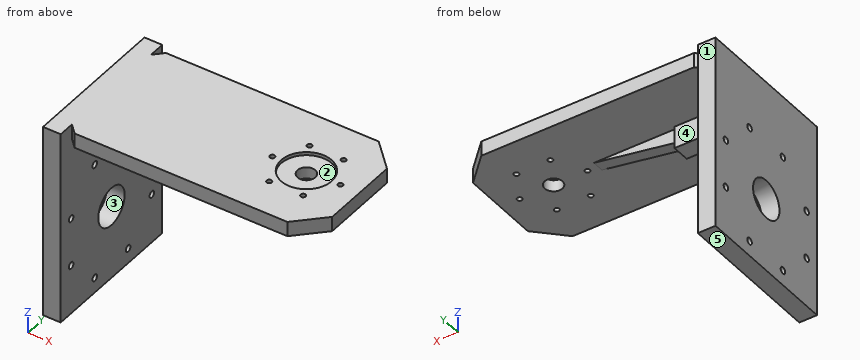
from build123d import *

# Parameters (mm, degrees)
SK_TOP_PLATE_R         = 1.7
SK_TOP_PLATE_R_2       = 6
TOP_PLATE_DEPTH        = 10
SK_YAW_PILOT_RECESS_R  = 17.15
YAW_PILOT_RECESS_DEPTH = 2.2
SK_BACK_PLATE_W        = 132
SK_BACK_PLATE_H        = 100
SK_BACK_PLATE_R        = 2.25
SK_BACK_PLATE_R_2      = 13
BACK_PLATE_DEPTH       = 12
RIB_DEPTH              = 8
SK_KEEL_W              = 58
SK_KEEL_H              = 15
KEEL_DEPTH             = 12


with BuildPart() as part:
    # SK_Top_Plate → Top_Plate (new body)
    with BuildSketch(Plane.XY.offset(72)):
        Polygon((-126, -45), (18, -45), (36, -27), (36, 27), (18, 45), (-126, 45), (-144, 27), (-144, -27), align=None)
        with Locations((23, 0)):
            Circle(SK_TOP_PLATE_R, mode=Mode.SUBTRACT)
        with Locations((11.5, 19.918584287)):
            Circle(SK_TOP_PLATE_R, mode=Mode.SUBTRACT)
        with Locations((-11.5, 19.918584287)):
            Circle(SK_TOP_PLATE_R, mode=Mode.SUBTRACT)
        with Locations((-23, 0)):
            Circle(SK_TOP_PLATE_R, mode=Mode.SUBTRACT)
        with Locations((-11.5, -19.918584287)):
            Circle(SK_TOP_PLATE_R, mode=Mode.SUBTRACT)
        with Locations((11.5, -19.918584287)):
            Circle(SK_TOP_PLATE_R, mode=Mode.SUBTRACT)
        Circle(SK_TOP_PLATE_R_2, mode=Mode.SUBTRACT)
    extrude(amount=TOP_PLATE_DEPTH)

    # SK_Yaw_Pilot_Recess → Yaw_Pilot_Recess (cut)
    with BuildSketch(Plane.XY.offset(82)):
        Circle(SK_YAW_PILOT_RECESS_R)
    extrude(amount=-YAW_PILOT_RECESS_DEPTH, mode=Mode.SUBTRACT)

    # SK_Back_Plate → Back_Plate (add)
    with BuildSketch(Plane(origin=(-144, 0, 0), x_dir=(0, 0, -1), z_dir=(1, 0, 0))):
        with Locations((-16, 0)):
            Rectangle(SK_BACK_PLATE_W, SK_BACK_PLATE_H)
        with Locations((39.726819898, 16.455387592)):
            Circle(SK_BACK_PLATE_R, mode=Mode.SUBTRACT)
        with Locations((16.455387592, 39.726819898)):
            Circle(SK_BACK_PLATE_R, mode=Mode.SUBTRACT)
        with Locations((-16.455387592, 39.726819898)):
            Circle(SK_BACK_PLATE_R, mode=Mode.SUBTRACT)
        with Locations((-39.726819898, 16.455387592)):
            Circle(SK_BACK_PLATE_R, mode=Mode.SUBTRACT)
        with Locations((-39.726819898, -16.455387592)):
            Circle(SK_BACK_PLATE_R, mode=Mode.SUBTRACT)
        with Locations((-16.455387592, -39.726819898)):
            Circle(SK_BACK_PLATE_R, mode=Mode.SUBTRACT)
        with Locations((16.455387592, -39.726819898)):
            Circle(SK_BACK_PLATE_R, mode=Mode.SUBTRACT)
        with Locations((39.726819898, -16.455387592)):
            Circle(SK_BACK_PLATE_R, mode=Mode.SUBTRACT)
        Circle(SK_BACK_PLATE_R_2, mode=Mode.SUBTRACT)
    extrude(amount=BACK_PLATE_DEPTH)

    # SK_Rib → Rib (add)
    with BuildSketch(Plane(origin=(0, -4, 0), x_dir=(1, 0, 0), z_dir=(0, 1, 0))):
        Polygon((-144, -52), (-30, -72), (-144, -72), align=None)
    extrude(amount=RIB_DEPTH)

    # SK_Keel → Keel (add)
    with BuildSketch(Plane(origin=(0, -6, 0), x_dir=(1, 0, 0), z_dir=(0, 1, 0))):
        with Locations((-115, -64.5)):
            Rectangle(SK_KEEL_W, SK_KEEL_H)
    extrude(amount=KEEL_DEPTH)


solid = part.part
The model under review builds one solid part; all positions refer to its coordinate system, in mm. Face numbers are marked on the shaded views. A direction names the side the tool comes from. Round coordinates to 2 decimals unless told otherwise and drop trailing zeros. Order: outer loops, then holes, each group sorted by start corner. A loop starts at its lowest first (then second) coordinate and runs counter-clockwise, first axis right, second up. Notation, with made-up numbers: (23.25, 18) -> (39.25, 18) arc R36 cw to (39.25, 56) -> close; hole circle Ø4 at (-18, 7). An arc over 180 degrees is marked (long way). Write item = value, one per line. Start each with the question number.
Item 1: For the marked faces 1 and 2, list the 3-axis set-ups (+Z, -Z, +X, -X, +Y, -Y) from which the entire face can be reached by the end or side of a thin tool; tool diameter is ignored.
Item 2: Consider section C-C on y = 32.5. Write out the cut boundary in (x, z), plus the area to 3 significant figures.
Item 3: Mouldability with a two-part tool opening along Y and no side actions: class the marked faces 3, 4 and 5 as released by +Y, released by -Y, zero draft, split by the parting line, or undercut.
Item 4: Clearance check with flat-ended pins moving along their axes: pin 1 Ø10 at (x, y) = (2, 35.5) entering from -Z; pin 2 Ø5 at (x, z) = (-63, 65.5) entering from +Y; pin 3 Ø19 at (x, y) = (0, 0) entering from +Z. State where each tip first meets the part, or that it passes through.
Item 5: Consider section D-D on x = -109. Write out the cut boundary in (y, z).
Item 6: For line 1 along Y through (x, z) = (11.5, 74.75); line 2 along Y through (x, z) = (-11, 77); line 3 along Z through (x, y) = (-127.5, -36.5), list the stretches that pass through material, from the lowest coordinate up.
Item 7: Consider section B-B on z = 3.5. Write out the cut boundary in (x, y), plus the area to 3 significant figures.
Item 8: Consider section A-A on x = 0. Write out the cut boundary in (y, z), plus the area to 3 significant figures.
Conclusion:
q1.face_1 = +Z, -Z, +X, -X, +Y
q1.face_2 = +Z
q2.outline = (-144, -50) -> (-132, -50) -> (-132, 72) -> (30.5, 72) -> (30.5, 82) -> (-144, 82) -> close
q2.area = 3,210 mm2
q3.face_3 = undercut
q3.face_4 = released by +Y
q3.face_5 = zero draft
q4.pin_1 = 72
q4.pin_2 = 4
q4.pin_3 = 79.8
q5.outline = (-45, 72) -> (-6, 72) -> (-6, 57) -> (6, 57) -> (6, 72) -> (45, 72) -> (45, 82) -> (-45, 82) -> close
q6.line_1 = -45 to -21.62, -18.22 to 18.22, 21.62 to 45
q6.line_2 = -45 to -21.54, -18.29 to 18.29, 21.54 to 45
q6.line_3 = 72 to 82
q7.outline = (-144, -50) -> (-132, -50) -> (-132, -12.52) -> (-144, -12.52) -> close; (-144, 12.52) -> (-132, 12.52) -> (-132, 50) -> (-144, 50) -> close
q7.area = 900 mm2
q8.outline = (-45, 72) -> (-6, 72) -> (-6, 79.8) -> (-17.15, 79.8) -> (-17.15, 82) -> (-45, 82) -> close; (6, 72) -> (45, 72) -> (45, 82) -> (17.15, 82) -> (17.15, 79.8) -> (6, 79.8) -> close
q8.area = 731 mm2
